from build123d import *

# Parameters (mm, degrees)
F1_DEPTH = 63.5
F0_W     = 25.5753439546
F0_H     = 19.05
F2_DEPTH = 19.05
F3_DEPTH = 15.875
F5_R     = 6.35


with BuildPart() as f1:
    # F0 (on Front) → F1 (new body, symmetric)
    with BuildSketch(Plane.XZ):
        Polygon((-41.275, -9.525), (41.275, -9.525), (41.275, 9.525), (22.225, 9.525), (-41.275, 9.525), align=None)
    extrude(amount=F1_DEPTH, both=True)

    # F0 (on Front) → F2 (join, symmetric)
    with BuildSketch(Plane.XZ):
        with BuildLine():
            Line((22.225, 9.525), (41.275, 9.525))
            Line((41.275, 9.525), (41.275, 27.0694342772))
            ThreePointArc((41.275, 27.0694342772), (46.461113991, 38.8066971986), (58.6310114503, 42.8752))
            Line((58.6310114503, 42.8752), (60.325, 42.8752))
            Line((60.325, 42.8752), (60.325, 61.9252))
            Line((60.325, 61.9252), (59.3480038392, 61.9252))
            add(Edge.make_bspline(
                [(54.2917304748, 61.8772770762), (55.9757916155, 61.9197178462), (57.6618264754, 61.9358036226), (59.3480038392, 61.9252)],
                knots=[109.3105529677, 109.3105529677, 109.3105529677, 109.3105529677, 113.4494154311, 113.4494154311, 113.4494154311, 113.4494154311], degree=3))
            ThreePointArc((54.2917304748, 61.8772770762), (31.4636155895, 50.7330198237), (22.225, 27.0694342772))
            Line((22.225, 27.0694342772), (22.225, 9.525))
        make_face()
        with Locations((73.1126719773, 52.4002)):
            Rectangle(F0_W, F0_H)
    extrude(amount=F2_DEPTH, both=True)

    # F0 (on Front) → F3 (join)
    with BuildSketch(Plane.XZ):
        with BuildLine():
            add(Edge.make_bspline(
                [(-41.275, 9.525), (-33.2862530849, 41.2521209724), (9.8143756106, 60.7563835758), (54.2917304748, 61.8772770762)],
                knots=[0, 0, 0, 0, 109.3105529677, 109.3105529677, 109.3105529677, 109.3105529677], degree=3))
            Line((-41.275, 9.525), (22.225, 9.525))
            Line((22.225, 9.525), (22.225, 27.0694342772))
            ThreePointArc((22.225, 27.0694342772), (31.4636155895, 50.7330198237), (54.2917304748, 61.8772770762))
        make_face()
    extrude(amount=F3_DEPTH)

    # F0 (on Front) → F4 (revolve)
    with BuildSketch(Plane.XZ):
        Polygon((85.9003439546, 61.9252), (85.9003439546, 42.8752), (85.9003439546, 38.1), (111.125, 38.1), (111.125, 66.675), (85.9003439546, 66.675), align=None)
    revolve(axis=Axis((85.9003439546, 0, 52.3875), (0, 0, 1)))

    # F5
    f5_edges = [f1.edges().sort_by_distance(p)[0] for p in [
        (-41.275, -63.5, 0),
        (41.275, -63.5, 0),
        (41.275, 63.5, 0),
        (-41.275, 63.5, 0),
    ]]
    fillet(f5_edges, radius=F5_R)


solid = f1.part
Work out the finished part from the listing and answer in its coordinate system (mm). A direction names the side the tool comes from. Round coordinates to 2 decimals unless told otherwise and drop trailing zeros. Write each loop counter-clockwise with the first axis right and the second up, starting at its lowest first coordinate (ties: lowest second). Pieces come first, ordered by that corner, then holes.
1) Straight lines are drawn through the part: line 1 (Z direction, x = -21, y = 35.5) (3 decimals); line 2 (Y direction, x = -0.5, z = 47) (3 decimals); line 3 (Z direction, x = 96.5, y = 8.5) (3 decimals). For each, find the intervals that lie inside material, in ascending order.
2) The mould has two halves that part along X. Classify faces 5 (the flat face through (22.225, 9, 18)), 6 (the cylindrical face through (39.464, -61.59, 0.133)), 7 (the flat face through (-1, -1, -9.525)), 8 (the cylindrical face through (46.325, -0.267, 38.681)): pulls with the +X half, pulls with the -X half, needs draft (parallel to the pull), parting line crosses it, or undercut.
3) Given pin 1 Ø8 at (x, z) = (14, 51.5) entering from +Y; pin 2 Ø4 at (x, y) = (-15.5, -7) entering from +Z; pin 3 Ø11 at (y, z) = (23.5, 7) entering from +X (3 decimals), each flat-ended and moving along its own axis, determine where each tip first touches the part or whether it passes through.
4) A tool of negligible diameter and unlimited length cuts with its end or side. For faces 1 (the flat face through (41.275, -1, 4)), 2 (the flat face through (60, 0, 61.925)), 3 (the flat face through (-3, 0, 30)), 4 (the flat face through (40, -19.05, 36)), from which of +Z, -Z, +X, -X, +Y, -Y can it reach the whole face along a straight path? Write none if from no direction.
5) A cutting plane is placed at A-A (z = 7). Give the vertices of the cut face in (x, y) (3 decimals), plus the area to 3 significant figures.
6) A cutting plane is placed at B-B (y = -34). Give the vertices of the cut face in (x, z) (3 decimals).
Completed:
1. line 1: z = -9.525 to 9.525
1. line 2: y = -15.875 to 0
1. line 3: z = 38.1 to 66.675
2. face 5: pulls with the -X half
2. face 6: pulls with the +X half
2. face 7: needs draft
2. face 8: undercut
3. pin 1: stops at y = 0
3. pin 2: stops at z = 43.6
3. pin 3: stops at x = 41.275
4. face 1: -Z, +X, +Y, -Y
4. face 2: +Z, -X
4. face 3: +Z, -X, +Y
4. face 4: +Z, -X, -Y
5. outline: (-41.275, -57.15) arc R6.35 ccw to (-34.925, -63.5) - (34.925, -63.5) arc R6.35 ccw to (41.275, -57.15) - (41.275, 57.15) arc R6.35 ccw to (34.925, 63.5) - (-34.925, 63.5) arc R6.35 ccw to (-41.275, 57.15) - close
5. area: 10,400 mm2
6. outline: (-41.275, -9.525) - (41.275, -9.525) - (41.275, 9.525) - (-41.275, 9.525) - close
